from build123d import *

# Parameters (mm, degrees)
EXTRUDE_1_DEPTH     = 1.5
EXTRUDE_2_DEPTH     = 4.5
SKETCH_5_R          = 24.25
EXTRUDE_4_DEPTH     = 3
EXTRUDE_5_DEPTH     = 1.5
SKETCH_7_R          = 0.5
CUT_EXTRUDE_2_DEPTH = 37.482872694
SKETCH_8_R          = 0.8
CUT_EXTRUDE_3_DEPTH = 4
SKETCH_9_R          = 1.1
CUT_EXTRUDE_4_DEPTH = 10


with BuildPart() as part:
    # 草图1 → 凸台-拉伸1 (new body)
    with BuildSketch(Plane.XY):
        with BuildLine():
            ThreePointArc((-18.273956879, 12.25), (0, 22), (18.273956879, 12.25))
            ThreePointArc((18.273956879, 12.25), (21.047886489, 6.402067973), (22, 0))
            Line((22, 0), (25, 0))
            ThreePointArc((25, 0), (0, 25), (-25, 0))
            Line((-25, 0), (-22, 0))
            ThreePointArc((-22, 0), (-21.047886489, 6.402067973), (-18.273956879, 12.25))
        make_face()
        with BuildLine():
            Line((25, 0), (22, 0))
            ThreePointArc((22, 0), (21.047886489, -6.402067973), (18.273956879, -12.25))
            ThreePointArc((18.273956879, -12.25), (0, -22), (-18.273956879, -12.25))
            ThreePointArc((-18.273956879, -12.25), (-21.047886489, -6.402067973), (-22, 0))
            Line((-22, 0), (-25, 0))
            ThreePointArc((-25, 0), (0, -25), (25, 0))
        make_face()
        with BuildLine():
            ThreePointArc((-18.273956879, -12.25), (0, -22), (18.273956879, -12.25))
            Line((18.273956879, -12.25), (11.787175234, -12.25))
            ThreePointArc((11.787175234, -12.25), (0, -17), (-11.787175234, -12.25))
            Line((-11.787175234, -12.25), (-18.273956879, -12.25))
        make_face()
        with BuildLine():
            Line((11.787175234, 12.25), (18.273956879, 12.25))
            ThreePointArc((18.273956879, 12.25), (0, 22), (-18.273956879, 12.25))
            Line((-18.273956879, 12.25), (-11.787175234, 12.25))
            ThreePointArc((-11.787175234, 12.25), (0, 17), (11.787175234, 12.25))
        make_face()
    extrude(amount=EXTRUDE_1_DEPTH)

    # 草图2 → 凸台-拉伸2 (add)
    with BuildSketch(Plane.XY.offset(1.5)):
        with BuildLine():
            Line((-18.903372715, 13.45), (-12.261219352, 13.45))
            ThreePointArc((-12.261219352, 13.45), (0, 18.2), (12.261219352, 13.45))
            Line((12.261219352, 13.45), (18.903372715, 13.45))
            ThreePointArc((18.903372715, 13.45), (23.2, 0), (18.903372715, -13.45))
            Line((18.903372715, -13.45), (12.261219352, -13.45))
            ThreePointArc((12.261219352, -13.45), (0, -18.2), (-12.261219352, -13.45))
            Line((-12.261219352, -13.45), (-18.903372715, -13.45))
            ThreePointArc((-18.903372715, -13.45), (-23.2, 0), (-18.903372715, 13.45))
        make_face()
        with BuildLine():
            Line((-18.273956879, 12.25), (-11.787175234, 12.25))
            ThreePointArc((-11.787175234, 12.25), (0, 17), (11.787175234, 12.25))
            Line((11.787175234, 12.25), (18.273956879, 12.25))
            ThreePointArc((18.273956879, 12.25), (22, 0), (18.273956879, -12.25))
            Line((18.273956879, -12.25), (11.787175234, -12.25))
            ThreePointArc((11.787175234, -12.25), (0, -17), (-11.787175234, -12.25))
            Line((-11.787175234, -12.25), (-18.273956879, -12.25))
            ThreePointArc((-18.273956879, -12.25), (-22, 0), (-18.273956879, 12.25))
        make_face(mode=Mode.SUBTRACT)
    extrude(amount=EXTRUDE_2_DEPTH)

    # 草图5 → 凸台-拉伸4 (add)
    with BuildSketch(Plane(origin=(0, 0, 0), x_dir=(-1, 0, 0), z_dir=(0, 0, -1))):
        Circle(SKETCH_5_R)
        with BuildLine():
            Line((-18.799933511, -13.25), (-12.183492931, -13.25))
            ThreePointArc((-12.183492931, -13.25), (0, -18), (12.183492931, -13.25))
            Line((12.183492931, -13.25), (18.799933511, -13.25))
            ThreePointArc((18.799933511, -13.25), (23, 0), (18.799933511, 13.25))
            Line((18.799933511, 13.25), (12.183492931, 13.25))
            ThreePointArc((12.183492931, 13.25), (0, 18), (-12.183492931, 13.25))
            Line((-12.183492931, 13.25), (-18.799933511, 13.25))
            ThreePointArc((-18.799933511, 13.25), (-23, 0), (-18.799933511, -13.25))
        make_face(mode=Mode.SUBTRACT)
    extrude(amount=EXTRUDE_4_DEPTH)

    # 草图6 → 凸台-拉伸5 (add)
    with BuildSketch(Plane.XY):
        with BuildLine():
            Line((-17, 24), (-17, 16.941074346))
            ThreePointArc((-17, 16.941074346), (-9.203646443, 22.16512784), (0, 24))
            Line((0, 24), (-17, 24))
        make_face()
        with BuildLine():
            ThreePointArc((0, 24), (9.203646443, 22.16512784), (17, 16.941074346))
            Line((17, 16.941074346), (17, 24))
            Line((17, 24), (0, 24))
        make_face()
        with BuildLine():
            ThreePointArc((17, -16.941074346), (9.203646443, -22.16512784), (0, -24))
            Line((0, -24), (17, -24))
            Line((17, -24), (17, -16.941074346))
        make_face()
        with BuildLine():
            Line((-17, -16.941074346), (-17, -24))
            Line((-17, -24), (0, -24))
            ThreePointArc((0, -24), (-9.203646443, -22.16512784), (-17, -16.941074346))
        make_face()
    extrude(amount=EXTRUDE_5_DEPTH)

    # 草图7 → 切除-拉伸2 (cut, through all)
    with BuildSketch(Plane(origin=(0, 0, -3), x_dir=(-1, 0, 0), z_dir=(0, 0, -1))):
        with Locations((-12.857243394, -14.660876246)):
            Circle(SKETCH_7_R)
        with Locations((-10.833619544, -16.21365744)):
            Circle(SKETCH_7_R)
        with Locations((-8.624629459, -17.48901846)):
            Circle(SKETCH_7_R)
        with Locations((-6.268069573, -18.465137525)):
            Circle(SKETCH_7_R)
        with Locations((-3.804261279, -19.125312968)):
            Circle(SKETCH_7_R)
        with Locations((-1.27536102, -19.458249003)):
            Circle(SKETCH_7_R)
        with Locations((1.27536102, -19.458249003)):
            Circle(SKETCH_7_R)
        with Locations((3.804261279, -19.125312968)):
            Circle(SKETCH_7_R)
        with Locations((6.268069573, -18.465137525)):
            Circle(SKETCH_7_R)
        with Locations((8.624629459, -17.48901846)):
            Circle(SKETCH_7_R)
    extrude(amount=-CUT_EXTRUDE_2_DEPTH, mode=Mode.SUBTRACT)

    # 草图8 → 切除-拉伸3 (cut)
    with BuildSketch(Plane.XY.offset(1.5)):
        with Locations((12.857243394, -14.660876246)):
            Circle(SKETCH_8_R)
        with Locations((10.833619544, -16.21365744)):
            Circle(SKETCH_8_R)
        with Locations((8.624629459, -17.48901846)):
            Circle(SKETCH_8_R)
        with Locations((6.268069573, -18.465137525)):
            Circle(SKETCH_8_R)
        with Locations((3.804261279, -19.125312968)):
            Circle(SKETCH_8_R)
        with Locations((1.27536102, -19.458249003)):
            Circle(SKETCH_8_R)
        with Locations((-1.27536102, -19.458249003)):
            Circle(SKETCH_8_R)
        with Locations((-3.804261279, -19.125312968)):
            Circle(SKETCH_8_R)
        with Locations((-6.268069573, -18.465137525)):
            Circle(SKETCH_8_R)
        with Locations((-8.624629459, -17.48901846)):
            Circle(SKETCH_8_R)
    extrude(amount=-CUT_EXTRUDE_3_DEPTH, mode=Mode.SUBTRACT)

    # 草图9 → 切除-拉伸4 (cut)
    with BuildSketch(Plane.XY.offset(1.5)):
        with Locations((-15, 22)):
            Circle(SKETCH_9_R)
        with Locations((15, -22)):
            Circle(SKETCH_9_R)
    extrude(amount=-CUT_EXTRUDE_4_DEPTH, mode=Mode.SUBTRACT)


solid = part.part
Model file for the job. Use its own axes, mm. A direction names the side the tool comes from. Coordinates: 2 decimals unless noted, no trailing zeros. Write each loop counter-clockwise with the first axis right and the second up, starting at its lowest first coordinate (ties: lowest second). Pieces come first, ordered by that corner, then holes. Notation, with made-up numbers: (-36.75, -2.5) - (-7.75, -2.5) arc R19 ccw to (-7.75, 25.5) - close; hole circle Ø5 at (65, -32). An arc over 180 degrees is marked (long way). Write each question's results on one line, items separated by ' | '. Start each with the question number.
1) Mould opens along Y. For faces 1 (the face through (-17, -21, 1)), 2 (the face through (-12, 24, 1)), 3 (the face through (15, 12.25, 3)), 4 (the face through (-23.2, -0.2, 3.7)) say: pulls with the +Y half, pulls with the -Y half, needs draft (parallel to the pull), parting line crosses it, or undercut.
2) 3-axis set-ups, long thin cutter, end or side, ignore diameter. For faces 5 (the face through (17, 21, 1)), 6 (the face through (17, -21, 1)), 7 (the face through (-12, -24, 1)), 8 (the face through (23, 0, -1)), 9 (the face through (-15, 12.25, 3)): which of +Z, -Z, +X, -X, +Y, -Y reach the whole face in a straight line?
3) Cut at B-B (x = -15). Write the cut outline in (y, z), then the cut area to 3 significant figures.
4) Flat gauge pins, fed straight in: P1, Ø4, axis at x = -11.5, z = 5, coming from the -Y side; P2, Ø1.3, axis at x = 1.28, y = -19.46, coming from the +Z side; P3, Ø4, axis at x = 11.5, z = 5, coming from the +Y side; P4, Ø3, axis at x = -3.5, y = 15, coming from the -Z side. Where does each tip first touch, or does it go through?
5) Cut at D-D (x = 14.5). Write the cut outline in (y, z), then the cut area to 3 significant figures.
6) Cut at A-A (z = 2.75). Write the cut outline in (x, y).
7) Cut at C-C (y = -9). Write the cut outline in (x, z), then the cut area to 3 significant figures.
8) Probe line 1 along Z through (x, y) = (0, -18.5); line 2 along Y through (x, z) = (-6, -1.25); line 3 along X through (y, z) = (8.5, 3.25). List the from-to ranges inside material, lowest first. Write a range as from..to.
Returned:
1) face 1: needs draft | face 2: pulls with the +Y half | face 3: undercut | face 4: parting line crosses it
2) face 5: +Z, -Z, +X, +Y | face 6: +Z, -Z, +X, -Y | face 7: +Z, -Z, -X, -Y | face 8: -Z | face 9: +Z, -Z
3) outline: (-24, 0) - (-19.05, 0) - (-19.05, -3) - (-13.25, -3) - (-13.25, 0) - (-12.25, 0) - (-12.25, 6) - (-13.45, 6) - (-13.45, 1.5) - (-24, 1.5) - close; (12.25, 0) - (13.25, 0) - (13.25, -3) - (19.05, -3) - (19.05, 0) - (20.9, 0) - (20.9, 1.5) - (13.45, 1.5) - (13.45, 6) - (12.25, 6) - close; (23.1, 0) - (24, 0) - (24, 1.5) - (23.1, 1.5) - close | area: 77.6 mm^2
4) P1: y = -15.52 | P2: z = -2.5 | P3: y = 15.52 | P4: through
5) outline: (-24, 0) - (-22.98, 0) - (-22.98, 1.5) - (-24, 1.5) - close; (-21.02, 0) - (-19.44, 0) - (-19.44, -3) - (-13.25, -3) - (-13.25, 0) - (-12.25, 0) - (-12.25, 6) - (-13.45, 6) - (-13.45, 1.5) - (-21.02, 1.5) - close; (12.25, 0) - (13.25, 0) - (13.25, -3) - (19.44, -3) - (19.44, 0) - (24, 0) - (24, 1.5) - (13.45, 1.5) - (13.45, 6) - (12.25, 6) - close | area: 80.2 mm^2
6) outline: (-18.9, -13.45) - (-12.26, -13.45) arc R18.2 ccw to (12.26, -13.45) - (18.9, -13.45) arc R23.2 ccw to (18.9, 13.45) - (12.26, 13.45) arc R18.2 ccw to (-12.26, 13.45) - (-18.9, 13.45) arc R23.2 ccw to start; hole (-18.27, -12.25) - (-11.79, -12.25) arc R17 ccw to (11.79, -12.25) - (18.27, -12.25) arc R22 ccw to (18.27, 12.25) - (11.79, 12.25) arc R17 ccw to (-11.79, 12.25) - (-18.27, 12.25) arc R22 ccw to start
7) outline: (-23.32, 0) - (-22.52, 0) - (-22.52, -3) - (-21.17, -3) - (-21.17, 0) - (-20.07, 0) - (-20.07, 6) - (-21.38, 6) - (-21.38, 1.5) - (-23.32, 1.5) - close; (20.07, 0) - (21.17, 0) - (21.17, -3) - (22.52, -3) - (22.52, 0) - (23.32, 0) - (23.32, 1.5) - (21.38, 1.5) - (21.38, 6) - (20.07, 6) - close | area: 29.6 mm^2
8) line 1: -3..1.5 | line 2: -23.5..-19.22, -17.71..-16.97, 16.97..23.5 | line 3: -21.59..-20.29, 20.29..21.59
